from build123d import *


with BuildPart() as part:
    # Sketch002 → Revolution (revolve)
    with BuildSketch(Plane.YZ):
        Polygon((1.6, 13), (1.6, 9.5), (3, 9.5), (3, 0), (17, 0), (17, 5.5), (3, 13), align=None)
    revolve(axis=Axis((0, 0, 0), (0, 0, 1)))


solid = part.part
The listing builds one solid part. Answer for the finished solid, in the listing's coordinates (mm). A direction names the side the tool comes from. Give positions to 0.01 mm unless a question says otherwise; leave off trailing zeros. Write each loop counter-clockwise with the first axis right and the second up, starting at its lowest first coordinate (ties: lowest second). Pieces come first, ordered by that corner, then holes. Notation, with made-up numbers: (-6, 33.5) - (47, 33.5) arc R22 cw to (47, 68.5) - close; hole circle Ø9 at (1.25, 36). An arc over 180 degrees is marked (long way). Use a Markdown table: item, result.
1. Section C-C on z = 2.5 is taken. Write down the section's boundary in (x, y), plus the area to 3 significant figures.
Values follow:
| item | result |
|---|---|
| outline | circle Ø34 at (0, 0); hole circle Ø6 at (0, 0) |
| area | 880 mm² |
2. Section D-D on z = 10.25 is taken. Write down the section's boundary in (x, y).
Values follow:
| item | result |
|---|---|
| outline | circle Ø16.27 at (0, 0); hole circle Ø3.2 at (0, 0) |
3. Each of these flat-tipped pins is pushed along its axis until it touches: P1, Ø5, axis at x = 0, y = 0, coming from the -Z side; P2, Ø1, axis at y = 1, z = 7, coming from the -X side; P3, Ø4, axis at x = -8, z = 8, coming from the -Y side. Where does it stop, or does it pass through?
Values follow:
| item | result |
|---|---|
| P1 | stops at z = 9.5 |
| P2 | stops at x = -15.1 |
| P3 | stops at y = -14.07 |
4. Section A-A on y = 0 is taken. Write down the section's boundary in (x, z).
Values follow:
| item | result |
|---|---|
| outline | (-17, 0) - (-3, 0) - (-3, 9.5) - (-1.6, 9.5) - (-1.6, 13) - (-3, 13) - (-17, 5.5) - close; (1.6, 9.5) - (3, 9.5) - (3, 0) - (17, 0) - (17, 5.5) - (3, 13) - (1.6, 13) - close |
5. Find the intervals of material crossed by probe 1 along X at (y, z) = (0, 4.75); probe 2 along Z at (x, y) = (2.5, 0); probe 3 along Y at (x, z) = (2, 6), in increasing order. Write a range as from..to.
Values follow:
| item | result |
|---|---|
| probe 1 | x = -17..-3, 3..17 |
| probe 2 | z = 9.5..13 |
| probe 3 | y = -15.94..-2.24, 2.24..15.94 |
6. For a pull along Y with two mould halves and no side action, classify faces 3 (the cylindrical face through (-14.334, 9.139, 2.788)), 4 (the cylindrical face through (0.97, -1.27, 11.23)), 5 (the flat face through (1.3, -1.3, 9.5)), 6 (the flat face through (1.3, 1.3, 13)) as released by +Y, released by -Y, zero draft, split by the parting line, or undercut.
Values follow:
| item | result |
|---|---|
| face 3 | split by the parting line |
| face 4 | undercut |
| face 5 | undercut |
| face 6 | zero draft |
7. A tool of negligible diameter and unlimited length cuts with its end or side. For faces 1 (the cylindrical face through (0, -3, 5)), 2 (the conical face through (1.409, 3.399, 12.636)), from which of +Z, -Z, +X, -X, +Y, -Y can it reach the whole face along a straight path? Write none if from no direction.
Values follow:
| item | result |
|---|---|
| face 1 | -Z |
| face 2 | +Z |
